Could you check a few things on this model? Use its own coordinates, in mm. Face numbers are marked on the shaded views. A direction names the side the tool comes from. Give positions to 0.01 mm unless a question says otherwise; leave off trailing zeros. Write each loop counter-clockwise with the first axis right and the second up, starting at its lowest first coordinate (ties: lowest second). Pieces come first, ordered by that corner, then holes. Notation, with made-up numbers: M 42.5,32 L 94.5,32 A10 cw 94.5,47 Z; hole C 61.5,-30 d1. An arc over 180 degrees is marked long. One line per item, written item: value.
```python
from build123d import *

# Parameters (mm, degrees)
F1_DEPTH = 7.62
F2_W     = 4.6228
F2_H     = 4.6228
F3_DEPTH = 86.106
F5_DEPTH = 25.4
F6_R     = 3.066051


with BuildPart() as f1:
    # F0 (on Top) → F1 (new body)
    with BuildSketch(Plane.XY):
        Polygon((-30.078946, 8.722895), (-30.078946, 23.962895), (33.675054, 23.962895), (33.675054, 8.722895), (35.961054, 8.722895), (35.961054, 26.248895), (-32.364946, 26.248895), (-32.364946, 8.722895), align=None)
    extrude(amount=F1_DEPTH)

    # F2 (on face) → F3 (cut)
    with BuildSketch(Plane.YZ.offset(35.961054)):
        with Locations((13.775022, 3.81)):
            Rectangle(F2_W, F2_H)
    extrude(amount=-F3_DEPTH, mode=Mode.SUBTRACT)

    # F4 (on face) → F5 (cut)
    with BuildSketch(Plane(origin=(0, 26.248895, 0), x_dir=(-1, 0, 0), z_dir=(0, 1, 0))):
        with BuildLine():
            Line((24.744946, 5.715), (-28.341054, 5.715))
            Line((-28.341054, 5.715), (-28.341054, 1.905))
            Line((-28.341054, 1.905), (24.744946, 1.905))
            ThreePointArc((24.744946, 1.905), (26.649946, 3.81), (24.744946, 5.715))
        make_face()
        with BuildLine():
            Line((-28.341054, 1.905), (-28.341054, 5.715))
            ThreePointArc((-28.341054, 5.715), (-30.246054, 3.81), (-28.341054, 1.905))
        make_face()
    extrude(amount=-F5_DEPTH, mode=Mode.SUBTRACT)

    # F6
    f6_edges = [f1.edges().sort_by_distance(p)[0] for p in [
        (35.961054, 26.248895, 3.81),
        (-32.364946, 26.248895, 3.81),
    ]]
    fillet(f6_edges, radius=F6_R)


solid = f1.part
```
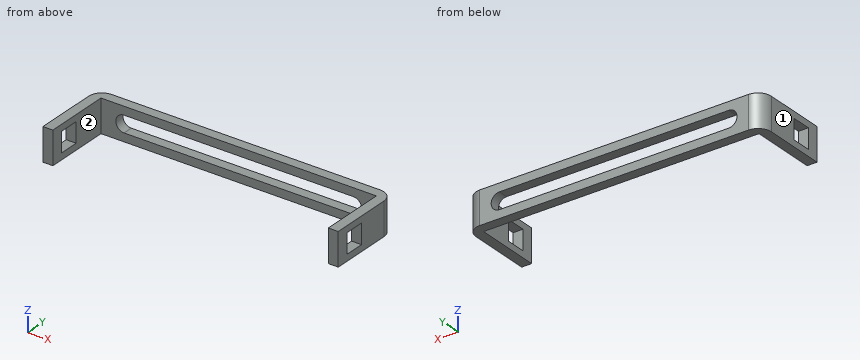
1) If we section it at B-B, the plane x = 7.5: Write out the boundary of the cut face in (y, z) (3 decimals), then the cut area to 3 significant figures.
Outcome:
outline: M 23.963,0 L 26.249,0 L 26.249,1.905 L 23.963,1.905 Z; M 23.963,5.715 L 26.249,5.715 L 26.249,7.62 L 23.963,7.62 Z
area: 8.71 mm^2
2) If we section it at A-A, the plane y = 15.5: Write out the boundary of the cut face in (x, z), then the cut area to 3 significant figures.
Outcome:
outline: M -32.36,0 L -30.08,0 L -30.08,1.5 L -32.36,1.5 Z; M -32.36,6.12 L -30.08,6.12 L -30.08,7.62 L -32.36,7.62 Z; M 33.68,0 L 35.96,0 L 35.96,1.5 L 33.68,1.5 Z; M 33.68,6.12 L 35.96,6.12 L 35.96,7.62 L 33.68,7.62 Z
area: 13.7 mm^2
3) On a 3-axis mill with a long thin cutter (end or side, diameter ignored), from which of +Z, -Z, +X, -X, +Y, -Y can I reach the whole of each face in a straight line? I mean the marked faces 1 and 2. Say none if no direction works.
Outcome:
face 1: +Z, -Z, -X, +Y, -Y
face 2: +Z, -Z, -Y
4) If we section it at C-C, the plane z = 3.81: Write out the boundary of the cut face in (x, y) (3 decimals), then the cut area to 3 significant figures.
Outcome:
outline: M -32.365,8.723 L -30.079,8.723 L -30.079,11.464 L -32.365,11.464 Z; M -32.365,16.086 L -30.079,16.086 L -30.079,23.963 L -26.65,23.963 L -26.65,26.249 L -29.299,26.249 A3.066 ccw -32.365,23.183 Z; M 30.246,23.963 L 33.675,23.963 L 33.675,16.086 L 35.961,16.086 L 35.961,23.183 A3.066 ccw 32.895,26.249 L 30.246,26.249 Z; M 33.675,8.723 L 35.961,8.723 L 35.961,11.464 L 33.675,11.464 Z
area: 70.6 mm^2
5) Please list where these lines run through material, in increasing order: L1, parallel to X at y = 23, z = 0.5; L2, parallel to Y at x = 4.5, z = 1.5; L3, parallel to X at y = 25.25, z = 5. Write a range as from..to.
Outcome:
L1: x = -32.36..-30.08, 33.68..35.96
L2: y = 23.96..26.25
L3: x = -31.56..-26.23, 29.83..35.16
6) I'm going to push flat-ended pins straight in: pin 1 (4 mm diameter, centred on x = -13.5, z = 6.5, fed in from -Y); pin 2 (2.5 mm diameter, centred on x = -4.5, y = 25, fed in from -Z); pin 3 (1.5 mm diameter, centred on x = -15.5, z = 3.5, fed in from +Y); pin 4 (0.7 mm diameter, centred on x = -30.5, z = 5, fed in from +Y). Where does each tip first touch, or does it pass through?
Outcome:
pin 1: stops at y = 23.96
pin 2: stops at z = 0
pin 3: passes through
pin 4: stops at y = 26.13
7) If we section it at D-D, the plane x = 31: Write out the boundary of the cut face in (y, z), then the cut area to 3 significant figures.
Outcome:
outline: M 23.96,0 L 26.25,0 L 26.25,7.62 L 23.96,7.62 Z
area: 17.4 mm^2
